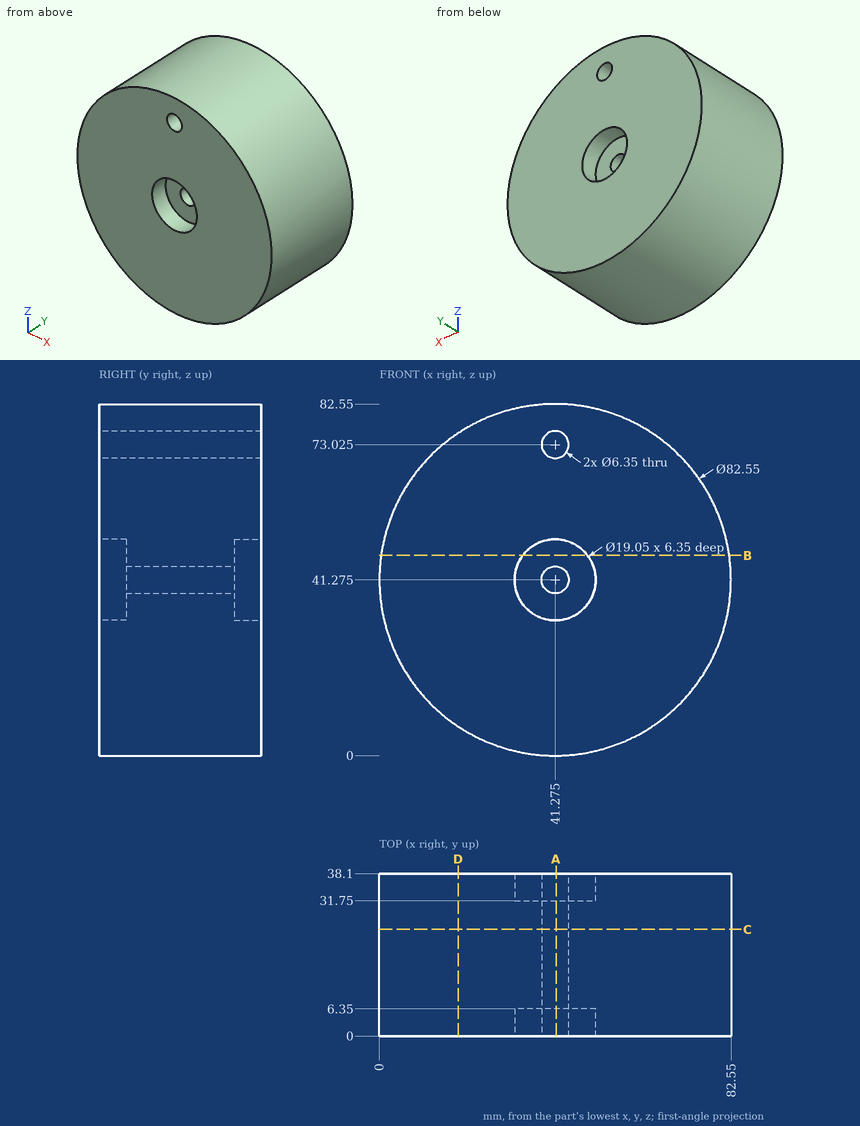
Design review of the part shown in the three views and the two pictorial views. Dimensions are in mm from the part's minimum x, y and z. Round coordinates to 2 decimals unless told otherwise and drop trailing zeros. Order: outer loops, then holes, each group sorted by start corner. A loop starts at its lowest first (then second) coordinate and runs counter-clockwise, first axis right, second up.
Item 1: Add section D-D, the plane x = 18.5. State the section outline as (y, z) points, and give its area (3 significant figures).
Working result:
outline: (0, 6.85) - (38.1, 6.85) - (38.1, 75.7) - (0, 75.7) - close
area: 2,620 mm2
Item 2: Add section A-A, the plane x = 41.5. State the section outline as (y, z) points.
Working result:
outline: (0, 0) - (38.1, 0) - (38.1, 31.75) - (31.75, 31.75) - (31.75, 38.11) - (6.35, 38.11) - (6.35, 31.75) - (0, 31.75) - close; (0, 50.8) - (6.35, 50.8) - (6.35, 44.44) - (31.75, 44.44) - (31.75, 50.8) - (38.1, 50.8) - (38.1, 69.86) - (0, 69.86) - close; (0, 76.19) - (38.1, 76.19) - (38.1, 82.55) - (0, 82.55) - close
Item 3: Add section B-B, the plane z = 47. State the section outline as (x, y) points.
Working result:
outline: (0.4, 0) - (33.66, 0) - (33.66, 6.35) - (48.89, 6.35) - (48.89, 0) - (82.15, 0) - (82.15, 38.1) - (48.89, 38.1) - (48.89, 31.75) - (33.66, 31.75) - (33.66, 38.1) - (0.4, 38.1) - close
Item 4: To check wall thickness, follow probe 1 along X at (y, z) = (26.5, 40.5); probe 2 along X at (y, z) = (3, 48); probe 3 along X at (y, z) = (18.5, 67). State the ranges of each line that lie inside material, in increasing order.
Working result:
probe 1: x = 0.01 to 38.2, 44.35 to 82.54
probe 2: x = 0.55 to 34.53, 48.02 to 82
probe 3: x = 9 to 73.55
Item 5: Add section C-C, the plane y = 25. State the section outline as (x, z) points (3 decimals).
Working result:
outline: circle Ø82.55 at (41.275, 41.275); hole circle Ø6.35 at (41.275, 41.275); hole circle Ø6.35 at (41.275, 73.025)
Item 6: For pin 1 (10 mm diameter, centred on y = 15.5, z = 14, fed in from +X); pin 2 (10 mm diameter, centred on x = 41.275, z = 41.275, fed in from -Y); pin 3 (6 mm diameter, centred on x = 14.5, y = 21.5, fed in from -Z), all flat-tipped, find the tip position at first contact; note any pin that passes through.
Working result:
pin 1: stops at x = 76.02
pin 2: stops at y = 6.35
pin 3: stops at z = 7.54
